from build123d import *

# Parameters (mm, degrees)
SKETCH1_R               = 3.1623
BOSS_EXTRUDE1_DEPTH     = 11.0998
CUT_EXTRUDE1_DEPTH      = 1
CUT_EXTRUDE1_DEPTH_BACK = 12.0998
SKETCH3_R               = 6.35
BOSS_EXTRUDE2_DEPTH     = 90.297
FILLET1_R               = 1.27


with BuildPart() as part:
    # Sketch1 → Boss-Extrude1 (new body)
    with BuildSketch(Plane.XY):
        Circle(SKETCH1_R)
    extrude(amount=BOSS_EXTRUDE1_DEPTH)

    # Sketch2 → Cut-Extrude1 (cut, two sides)
    with BuildSketch(Plane(origin=(0, 0, 0), x_dir=(-1, 0, 0), z_dir=(0, 0, -1))) as cut_extrude1_sk:
        Polygon((17.073178183, -20.234228338), (0.001249598, -3.162299753), (-3.162299753, 0.001249598), (-20.234228338, 17.073178183), (-54.378085507, -17.070678986), (-17.070678986, -54.378085507), align=None)
    extrude(amount=CUT_EXTRUDE1_DEPTH, mode=Mode.SUBTRACT)
    extrude(cut_extrude1_sk.sketch, amount=-CUT_EXTRUDE1_DEPTH_BACK, mode=Mode.SUBTRACT)

    # Sketch3 → Boss-Extrude2 (add)
    with BuildSketch(Plane.XY.offset(11.0998)):
        Circle(SKETCH3_R)
    extrude(amount=BOSS_EXTRUDE2_DEPTH)

    # Fillet1
    fillet1_edges = [part.edges().sort_by_distance(p)[0] for p in [
        (-2.236083774, 2.236083774, 11.0998),
        (1.580525077, -1.580525077, 11.0998),
    ]]
    fillet(fillet1_edges, radius=FILLET1_R)


solid = part.part
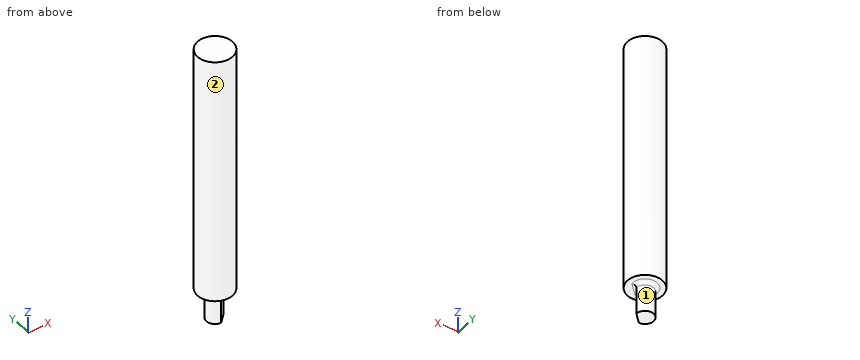
CAD build for the part. Positions are in the model's coordinates, mm. Face numbers are marked on the shaded views. A direction names the side the tool comes from. Give positions to 0.01 mm unless a question says otherwise; leave off trailing zeros. Write each loop counter-clockwise with the first axis right and the second up, starting at its lowest first coordinate (ties: lowest second). Pieces come first, ordered by that corner, then holes. Notation, with made-up numbers: (-7, 58) - (28, 58) arc R19 ccw to (28, 64) - close; hole circle Ø6 at (26, -5.5). An arc over 180 degrees is marked (long way). Put each result on its own line as item: value.
(1) Drop flat-ended pins along their axis: pin 1 Ø5 at (y, z) = (4.5, 59.5) entering from -X; pin 2 Ø3 at (x, z) = (-4, 49) entering from -Y. Give the stop position or say it passes through.
Working result:
pin 1: x = -6.03
pin 2: y = -5.84
(2) Wall check: L1, parallel to Z at x = -4.25, y = 3.5; L2, parallel to Y at x = -0.25, z = 21.5; L3, parallel to X at y = -5.5, z = 86.5. Give the ranges that are in metal, low to high.
Working result:
L1: 11.1 to 101.4
L2: -6.35 to 6.35
L3: -3.17 to 3.17
(3) Tool access for the marked faces 1 and 2: list every direction of +Z, -Z, +X, -X, +Y, -Y with a clear straight run to the whole face (end or side of a thin tool).
Working result:
face 1: -Z
face 2: +Z, -Z
(4) Saw through at B-B (x = -5.5). List the corners of the cut face in (y, z).
Working result:
outline: (-3.17, 11.1) - (3.17, 11.1) - (3.17, 101.4) - (-3.17, 101.4) - close
(5) Saw through at A-A (z = 76). List the corners of the cut face in (x, y), then the cut area to 3 significant figures.
Working result:
outline: circle Ø12.7 at (0, 0)
area: 127 mm^2
